The listing builds one solid part. Answer for the finished solid, in the listing's coordinates (mm). Face numbers are marked on the shaded views. A direction names the side the tool comes from. Coordinates: 2 decimals unless noted, no trailing zeros. Order: outer loops, then holes, each group sorted by start corner. A loop starts at its lowest first (then second) coordinate and runs counter-clockwise, first axis right, second up. Notation, with made-up numbers: (48, -5) -> (57, -5) arc R24 ccw to (57, 21) -> close; hole circle Ø2 at (68.25, -18). An arc over 180 degrees is marked (long way). Put each result on its own line as item: value. Start each with the question number.
```python
from build123d import *

# Parameters (mm, degrees)
SKETCH1_W           = 55
SKETCH1_H           = 65
BOSS_EXTRUDE1_DEPTH = 13
SKETCH2_W           = 25
SKETCH2_H           = 45
BOSS_EXTRUDE2_DEPTH = 50
SKETCH5_R           = 20.5
CUT_EXTRUDE1_DEPTH  = 20
SKETCH7_R           = 7
CUT_EXTRUDE2_DEPTH  = 20
SKETCH8_R           = 2.25
CUT_EXTRUDE3_DEPTH  = 20
FILLET1_R           = 10


with BuildPart() as part:
    # Sketch1 → Boss-Extrude1 (new body)
    with BuildSketch(Plane(origin=(0, 0, 0), x_dir=(1, 0, 0), z_dir=(0, 1, 0))):
        with Locations((-5, 0)):
            Rectangle(SKETCH1_W, SKETCH1_H)
    extrude(amount=BOSS_EXTRUDE1_DEPTH)

    # Sketch2 → Boss-Extrude2 (add)
    with BuildSketch(Plane(origin=(0, 13, 0), x_dir=(1, 0, 0), z_dir=(0, 1, 0))):
        with Locations((10, 0)):
            Rectangle(SKETCH2_W, SKETCH2_H)
    extrude(amount=BOSS_EXTRUDE2_DEPTH)

    # Sketch5 → Cut-Extrude1 (cut)
    with BuildSketch(Plane(origin=(22.5, 0, 0), x_dir=(0, 0, -1), z_dir=(1, 0, 0))):
        with Locations((0, 35)):
            Circle(SKETCH5_R)
    extrude(amount=-CUT_EXTRUDE1_DEPTH, mode=Mode.SUBTRACT)

    # Sketch7 → Cut-Extrude2 (cut)
    with BuildSketch(Plane(origin=(2.5, 0, 0), x_dir=(0, 0, -1), z_dir=(1, 0, 0))):
        with Locations((0, 35)):
            Circle(SKETCH7_R)
    extrude(amount=-CUT_EXTRUDE2_DEPTH, mode=Mode.SUBTRACT)

    # Sketch8 → Cut-Extrude3 (cut)
    with BuildSketch(Plane(origin=(0, 0, 0), x_dir=(-1, 0, 0), z_dir=(0, -1, 0))):
        with Locations(Location((12.5, -22.5, 0), (0, 0, 90))):
            Circle(SKETCH8_R)
        with Locations(Location((12.5, 22.5, 0), (0, 0, 90))):
            Circle(SKETCH8_R)
        with Locations(Location((-12.5, 22.5, 0), (0, 0, 90))):
            Circle(SKETCH8_R)
        with Locations(Location((-12.5, -22.5, 0), (0, 0, 90))):
            Circle(SKETCH8_R)
    extrude(amount=-CUT_EXTRUDE3_DEPTH, mode=Mode.SUBTRACT)

    # Fillet1
    fillet1_edges = [part.edges().sort_by_distance(p)[0] for p in [
        (-32.5, 6.5, -32.5),
    ]]
    fillet(fillet1_edges, radius=FILLET1_R)


solid = part.part
```
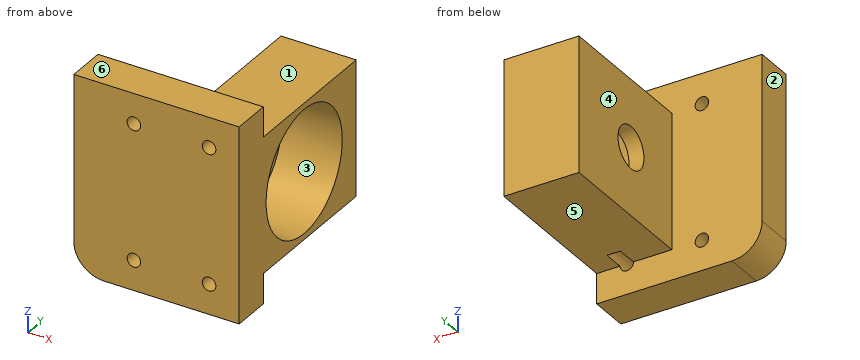
(1) For a pull along Z with two mould halves and no side action, classify the marked faces 1, 2 and 3 as released by +Z, released by -Z, zero draft, split by the parting line, or undercut.
(2) The part is cut by section D-D on z = 0. Determine the outline of the cut face in (x, y), plus the area to 4 significant figures.
(3) The part is cut by section B-B on x = -12.5. Determine the outline of the cut face in (y, z), plus the area to 3 significant figures.
(4) The part is cut by section A-A on x = 12.5. Determine the outline of the cut face in (y, z), plus the area to 3 significant figures.
(5) Find the intervals of material crossed by L1, parallel to X at y = 10.25, z = 22.5; L2, parallel to Z at x = -12, y = 7; L3, parallel to Y at x = 19, z = 0, in increasing order.
(6) The part is cut by section C-C on y = 35. Determine the outline of the cut face in (x, z), plus the area to 3 significant figures.
(7) Each of these flat-tipped pins is pushed along its axis until it touches: P1, Ø1, axis at x = -1.5, y = 17, coming from the -Z side; P2, Ø1.5, axis at x = -15, z = -1, coming from the +Y side; P3, Ø0.7, axis at x = 13.5, z = 21.5, coming from the -Y side. Where does it stop, or does it pass through?
(8) A tool of negligible diameter and unlimited length cuts with its end or side. For the marked faces 4, 5 and 6, from which of +Z, -Z, +X, -X, +Y, -Y can it reach the whole face along a straight path? Write none if from no direction.
Worked out:
1. face 1: released by +Z
1. face 2: zero draft
1. face 3: undercut
2. outline: (-32.5, 0) -> (22.5, 0) -> (22.5, 14.5) -> (2.5, 14.5) -> (2.5, 28) -> (-2.5, 28) -> (-2.5, 13) -> (-32.5, 13) -> close; (-2.5, 42) -> (2.5, 42) -> (2.5, 55.5) -> (22.5, 55.5) -> (22.5, 63) -> (-2.5, 63) -> close
2. area: 1,075 mm2
3. outline: (0, -32.5) -> (13, -32.5) -> (13, -24.75) -> (0, -24.75) -> close; (0, -20.25) -> (13, -20.25) -> (13, 20.25) -> (0, 20.25) -> close; (0, 24.75) -> (13, 24.75) -> (13, 32.5) -> (0, 32.5) -> close
3. area: 728 mm2
4. outline: (0, -32.5) -> (13, -32.5) -> (13, -24.75) -> (0, -24.75) -> close; (0, -20.25) -> (20, -20.25) -> (20, -22.5) -> (63, -22.5) -> (63, 22.5) -> (20, 22.5) -> (20, 20.25) -> (0, 20.25) -> close; (0, 24.75) -> (13, 24.75) -> (13, 32.5) -> (0, 32.5) -> close; hole circle Ø41 at (35, 0)
4. area: 1,630 mm2
5. L1: -32.5 to -14.75, -10.25 to 10.25, 14.75 to 22.5
5. L2: -32.5 to -24.69, -20.31 to 20.31, 24.69 to 32.5
5. L3: 0 to 14.5, 55.5 to 63
6. outline: (-2.5, -22.5) -> (22.5, -22.5) -> (22.5, -20.5) -> (2.5, -20.5) -> (2.5, -7) -> (-2.5, -7) -> close; (-2.5, 7) -> (2.5, 7) -> (2.5, 20.5) -> (22.5, 20.5) -> (22.5, 22.5) -> (-2.5, 22.5) -> close
6. area: 235 mm2
7. P1: z = -22.5
7. P2: y = 13
7. P3: y = 20
8. face 4: +Z, -Z, -X, +Y
8. face 5: -Z, +X, -X, +Y
8. face 6: +Z, +X, -X, +Y, -Y
